from build123d import *

# Parameters (mm, degrees)
F0_W     = 86
F0_H     = 73
F1_DEPTH = 25
F2_T     = -2.5


with BuildPart() as f1:
    # F0 (on Right) → F1 (new body)
    with BuildSketch(Plane.YZ):
        Rectangle(F0_W, F0_H)
    extrude(amount=F1_DEPTH)

    # F2
    f2_openings = [f1.faces().sort_by_distance(p)[0] for p in [
        (25, 0, 0),
    ]]
    offset(amount=F2_T, openings=f2_openings)


solid = f1.part
Input: part model. Units: mm. Frame: model coordinates. A direction names the side the tool comes from. Give positions to 0.01 mm unless a question says otherwise; leave off trailing zeros. Loops run counter-clockwise (first coordinate to the right, second up) from the corner with the lowest first, then second, coordinate; pieces in that order, holes last. Notation, with made-up numbers: (55.5, 10.25) - (109.5, 10.25) arc R23 cw to (109.5, 18.25) - close; hole circle Ø2 at (8.25, 51.25). An arc over 180 degrees is marked (long way). Use CSV: the item, a comma, the result in double quotes. Start each with the question number.
Item 1: Reachability of faces 4 (the flat face through (12, -1, -36.5)), 5 (the flat face through (14, 40.5, 0)) from +Z, -Z, +X, -X, +Y, -Y: full face, straight path, thin tool, end or side. Return the list, or none.
Item 2: Section C-C on y = 35. Return loops of the section in (x, z), then the cut area to 3 significant figures.
Item 3: Contact query for a flat-ended pin moving along its axis: P1, Ø1.5, axis at y = 11, z = 15.5, coming from the +X side. Output: stop coordinate, or through.
Item 4: Mould query, pull axis Y, two halves, no side actions, for faces 1 (the flat face through (12, 43, -1)), 2 (the flat face through (14, -40.5, 0)), 3 (the flat face through (25, -3, -35)). Classes: pulls with the +Y half, pulls with the -Y half, needs draft (parallel to the pull), parting line crosses it, or undercut.
Item 5: Section A-A on x = 23.25. Return loops of the section in (y, z).
Item 6: Section B-B on z = -14.5. Return loops of the section in (x, y).
Item 7: Line query: line 1 (Z direction, x = 23.25, y = 18); line 2 (Y direction, x = 5.5, z = -19); line 3 (X direction, y = -7, z = 17.5). Output: solid intervals per line, ascending.
Ans:
1,face 4,"-Z, +X, -X, +Y, -Y"
1,face 5,"+X"
2,outline,"(0, -36.5) - (25, -36.5) - (25, -34) - (2.5, -34) - (2.5, 34) - (25, 34) - (25, 36.5) - (0, 36.5) - close"
2,area,"295 mm2"
3,P1,"stops at x = 2.5"
4,face 1,"pulls with the +Y half"
4,face 2,"undercut"
4,face 3,"needs draft"
5,outline,"(-43, -36.5) - (43, -36.5) - (43, 36.5) - (-43, 36.5) - close; hole (-40.5, -34) - (40.5, -34) - (40.5, 34) - (-40.5, 34) - close"
6,outline,"(0, -43) - (25, -43) - (25, -40.5) - (2.5, -40.5) - (2.5, 40.5) - (25, 40.5) - (25, 43) - (0, 43) - close"
7,line 1,"z = -36.5 to -34, 34 to 36.5"
7,line 2,"y = -43 to -40.5, 40.5 to 43"
7,line 3,"x = 0 to 2.5"
